Build history of the part. All positions in model axes, mm. A direction names the side the tool comes from. Give positions to 0.01 mm unless a question says otherwise; leave off trailing zeros. Order: outer loops, then holes, each group sorted by start corner. A loop starts at its lowest first (then second) coordinate and runs counter-clockwise, first axis right, second up. Notation, with made-up numbers: (-30.5, -39) - (-1.5, -39) arc R13 ccw to (-1.5, -26) - close; hole circle Ø2 at (81.5, 17). An arc over 180 degrees is marked (long way). Write each question's results on one line, items separated by ' | '. Start each with the question number.
from build123d import *

# Parameters (mm, degrees)
F1_DEPTH      = 16
F1_DEPTH_BACK = 16


# Not quite as in the source:
# - a feature names something its author has since deleted; it is built from what else it names


with BuildPart() as f1:
    # F0 (on Front) → F1 (new body, two sides)
    with BuildSketch(Plane.XZ) as f1_sk:
        Polygon((-9, 77.4134680122), (-27, 77.4134680122), (-27, -272.5865319878), (-9, -272.5865319878), (9, -272.5865319878), (27, -272.5865319878), (27, 77.4134680122), (9, 77.4134680122), (9, -86.6605598913), (-9, -86.6605598913), align=None)
    extrude(amount=F1_DEPTH)
    extrude(f1_sk.sketch, amount=-F1_DEPTH_BACK)


solid = f1.part
Item 1: Two-plate mould, pull along X, no slides. Class faces 1 (the flat face through (-27, 0, -95)), 2 (the flat face through (0, 0, -272.587)), 3 (the flat face through (9, 0, -3)): +X half, -X half, draft (parallel to the pull), parting line (faces both ways), or undercut.
Item 2: Cut at A-A, the plane z = 0.5. List the corners of the cut face in (x, y), then the cut area to 3 significant figures.
Item 3: Probe line 1 along X through (y, z) = (-12.5, 19); line 2 along Z through (x, y) = (2.5, 5.5). List the from-to ranges inside material, lowest first. Write a range as from..to.
Item 4: Which spindle directions (+Z, -Z, +X, -X, +Y, -Y) get a long thin tool onto all of the face, cutting with end or side? Do faces 4 (the flat face through (-9, 0, -6)), 5 (the flat face through (0, -16, -95)). Say none if no direction does.
Item 5: Cut at B-B, the plane y = -3. List the corners of the cut face in (x, z).
Item 6: Flat gauge pins, fed straight in: pin 1 Ø8 at (x, z) = (-8.5, -20) entering from -Y; pin 2 Ø5 at (x, y) = (1.5, -5) entering from +Z. Where does each tip first touch, or does it go through?
Values found:
1) face 1: -X half | face 2: draft | face 3: undercut
2) outline: (-27, -16) - (-9, -16) - (-9, 16) - (-27, 16) - close; (9, -16) - (27, -16) - (27, 16) - (9, 16) - close | area: 1,150 mm2
3) line 1: x = -27..-9, 9..27 | line 2: z = -272.59..-86.66
4) face 4: +Z, +Y, -Y | face 5: +Z, -Z, +X, -X, -Y
5) outline: (-27, -272.59) - (27, -272.59) - (27, 77.41) - (9, 77.41) - (9, -86.66) - (-9, -86.66) - (-9, 77.41) - (-27, 77.41) - close
6) pin 1: stops at y = -16 | pin 2: stops at z = -86.66
